Drawing for the job (mm, zero at the part's lowest x, y, z). A direction names the side the tool comes from. Give positions to 0.01 mm unless a question says otherwise; leave off trailing zeros. Order: outer loops, then holes, each group sorted by start corner. A loop starts at its lowest first (then second) coordinate and runs counter-clockwise, first axis right, second up. Notation, with made-up numbers: (87, 14.25) -> (129, 14.25) arc R17 cw to (129, 28.25) -> close; hole circle Ø1 at (50.25, -14). An arc over 180 degrees is marked (long way). One line per item, written item: value. Start each with the question number.
(1) Probe line 1 (Z direction, x = 16.5, y = 6); line 2 (Y direction, x = 19.5, z = 4.25); line 3 (Y direction, x = 20.5, z = 2.5) (1 decimal). List the from-to ranges inside material, lowest first.
(2) Saw through at B-B on y = 18. Give the cut face in (x, z) (1 decimal), plus the area to 3 significant figures.
(3) Pin check, flat tips, straight feed: pin 1 (3 mm diameter, centred on y = 12.5, z = 7, fed in from -X); pin 2 (2 mm diameter, centred on x = 8, z = 3.5, fed in from +Y); pin 3 (2 mm diameter, centred on y = 9.5, z = 4, fed in from -X). Stop position of each tip, or through.
(4) Which spindle directions (+Z, -Z, +X, -X, +Y, -Y) get a long thin tool onto all of the face, cutting with end or side? Do the marked faces 4 and 5. Say none if no direction does.
(5) Saw through at A-A on x = 14. Give the cut face in (y, z), plus the area to 3 significant figures.
(6) Saw through at C-C on x = 8.5. Give the cut face in (y, z), plus the area to 3 significant figures.
(7) Two-plate mould, pull along X, no slides. Class the marked faces 1, 2 and 3: +X half, -X half, draft (parallel to the pull), parting line (faces both ways), or undercut.
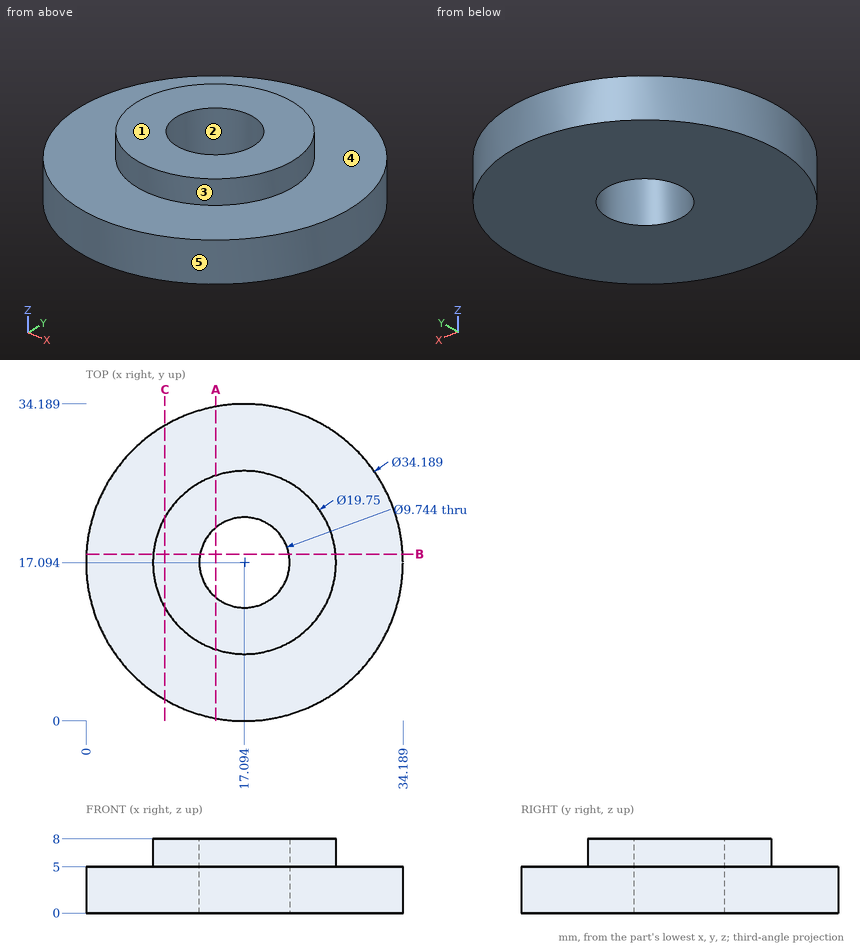
Results below:
1. line 1: z = 0 to 5
1. line 2: y = 0.17 to 12.86, 21.33 to 34.02
1. line 3: y = 0.3 to 13.6, 20.6 to 33.8
2. outline: (0, 0) -> (12.3, 0) -> (12.3, 8) -> (7.3, 8) -> (7.3, 5) -> (0, 5) -> close; (21.9, 0) -> (34.2, 0) -> (34.2, 5) -> (26.9, 5) -> (26.9, 8) -> (21.9, 8) -> close
2. area: 153 mm²
3. pin 1: stops at x = 7.72
3. pin 2: stops at y = 32.15
3. pin 3: stops at x = 1.32
4. face 4: +Z
4. face 5: +Z, -Z
5. outline: (0.28, 0) -> (13.33, 0) -> (13.33, 8) -> (7.72, 8) -> (7.72, 5) -> (0.28, 5) -> close; (20.86, 0) -> (33.91, 0) -> (33.91, 5) -> (26.47, 5) -> (26.47, 8) -> (20.86, 8) -> close
5. area: 164 mm²
6. outline: (2.32, 0) -> (31.87, 0) -> (31.87, 5) -> (21.96, 5) -> (21.96, 8) -> (12.23, 8) -> (12.23, 5) -> (2.32, 5) -> close
6. area: 177 mm²
7. face 1: draft
7. face 2: undercut
7. face 3: parting line
